```python
from build123d import *

# Parameters (mm, degrees)
F0_R     = 2.475
F0_R_2   = 1.69
F1_DEPTH = 1.33
F2_R     = 7.775
F3_DEPTH = 3.15
F4_R     = 3.215
F5_DEPTH = 2


with BuildPart() as f1:
    # F0 (on Front) → F1 (new body)
    with BuildSketch(Plane.XZ):
        Circle(F0_R)
        Circle(F0_R_2, mode=Mode.SUBTRACT)
    extrude(amount=F1_DEPTH)

    # F2 (on face) → F3 (join)
    with BuildSketch(Plane.XZ.offset(1.33)):
        Circle(F2_R)
    extrude(amount=F3_DEPTH)

    # F4 (on face) → F5 (cut)
    with BuildSketch(Plane.XZ.offset(4.48)):
        Circle(F4_R)
    extrude(amount=-F5_DEPTH, mode=Mode.SUBTRACT)


solid = f1.part
```
Geometry check sheet. Reference: the model listing, model coordinates, mm. A direction names the side the tool comes from. Coordinates: 2 decimals unless noted, no trailing zeros. Write each loop counter-clockwise with the first axis right and the second up, starting at its lowest first coordinate (ties: lowest second). Pieces come first, ordered by that corner, then holes. Notation, with made-up numbers: M 5.25,-2 L 64.25,-2 A34 cw 64.25,29 Z; hole C 70.5,89 d5. An arc over 180 degrees is marked long. Use one line per item in the form item = value. Start each with the question number.
1) Set-up check for faces 4 (the cylindrical face through (-2.55, -3.49, -1.96)), 5 (the cylindrical face through (2.36, -0.66, 0.74)), 6 (the flat face through (3, -4.48, -2)): record each of +Z, -Z, +X, -X, +Y, -Y from which the full face is reachable in a straight line by a thin tool's end or side.
2) Thickness scan on probe 1 along Z at (x, y) = (0, -3.1) (3 decimals); probe 2 along Z at (x, y) = (0, -0.5) (3 decimals); probe 3 along Y at (x, z) = (1.75, -2.25). Record the ranges inside material, lowest first. Write a range as from..to.
3) Section check A-A on x = 0. Enter the section's corners in (y, z) (3 decimals), and give its area (3 significant figures).
4) Section check C-C on y = -3. Enter the section's corners in (x, z) (3 decimals).
5) Release check for a two-part mould opening along Z. For faces 1 (the flat face through (0, -2.48, 0)), 2 (the cylindrical face through (-1.69, -2.88, -7.59)), 3 (the flat face through (-2, -1.33, 2)) record: pulls with the +Z half, pulls with the -Z half, needs draft (parallel to the pull), parting line crosses it, or undercut.
6) Section check D-D on z = 3. Enter the section's corners in (x, y), and give its area (3 significant figures).
7) Go/stop test with flat-tipped pins: pin 1 Ø3 at (x, z) = (-0.5, 1) entering from -Y; pin 2 Ø1.5 at (x, y) = (2, -1.5) entering from -Z; pin 3 Ø1.7 at (x, z) = (0.5, 0) entering from +Y. Record where each tip stops, or that it passes through.
8) Section check B-B on z = 0. Enter the section's corners in (x, y) (3 decimals), and give its area (3 significant figures).
Responses:
q1.face_4 = -Y
q1.face_5 = +Y
q1.face_6 = +Z, -Z, +X, -X, -Y
q2.probe_1 = -7.775..-3.215, 3.215..7.775
q2.probe_2 = -2.475..-1.69, 1.69..2.475
q2.probe_3 = -2.48..-1.33
q3.outline = M -4.48,-7.775 L -1.33,-7.775 L -1.33,-2.475 L 0,-2.475 L 0,-1.69 L -1.33,-1.69 L -1.33,1.69 L 0,1.69 L 0,2.475 L -1.33,2.475 L -1.33,7.775 L -4.48,7.775 L -4.48,3.215 L -2.48,3.215 L -2.48,-3.215 L -4.48,-3.215 Z
q3.area = 38.2 mm2
q4.outline = C 0,0 d15.55; hole C 0,0 d6.43
q5.face_1 = undercut
q5.face_2 = parting line crosses it
q5.face_3 = needs draft
q6.outline = M -7.17,-4.48 L -1.16,-4.48 L -1.16,-2.48 L 1.16,-2.48 L 1.16,-4.48 L 7.17,-4.48 L 7.17,-1.33 L -7.17,-1.33 Z
q6.area = 40.6 mm2
q7.pin_1 = -2.48
q7.pin_2 = -7.67
q7.pin_3 = -1.33
q8.outline = M -7.775,-4.48 L -3.215,-4.48 L -3.215,-2.48 L 3.215,-2.48 L 3.215,-4.48 L 7.775,-4.48 L 7.775,-1.33 L 2.475,-1.33 L 2.475,0 L 1.69,0 L 1.69,-1.33 L -1.69,-1.33 L -1.69,0 L -2.475,0 L -2.475,-1.33 L -7.775,-1.33 Z
q8.area = 38.2 mm2
